Source: CAD feature listing. Evaluate the final solid. Frame: model axes, mm. A direction names the side the tool comes from. Coordinates: 2 decimals unless noted, no trailing zeros. Order: outer loops, then holes, each group sorted by start corner. A loop starts at its lowest first (then second) coordinate and runs counter-clockwise, first axis right, second up.
Item 1: Contact query for flat-ended pins moving along their axis: P1, Ø5.5, axis at x = -20, y = 0, coming from the -Z side; P2, Ø1, axis at y = 7.5, z = 121.5, coming from the -X side; P3, Ø5, axis at x = 9.5, z = 38.5, coming from the -Y side; P4, Ø2.5, axis at x = 0, y = 0, coming from the -Z side. Output: stop coordinate, or through.
Item 2: Ray query, line 1 (Y direction, x = 0, z = 12); line 2 (Z direction, x = 11, y = 11); line 3 (X direction, y = -20, z = 20). Return the intervals inside material, ascending.
Item 3: Reachability of faces 1 (the flat face through (0, -4, -14)), 2 (the flat face through (5, -5, 0)), 3 (the flat face through (0, 0, 191)) from +Z, -Z, +X, -X, +Y, -Y: full face, straight path, thin tool, end or side. Return the list, or none.
Item 4: Mould query, pull axis X, two halves, no side actions, for faces 4 (the conical face through (0.08, 19.64, 33.04)), 5 (the cylindrical face through (-20.633, -15.821, 94.181)), 6 (the flat face through (1, 1, -22)). Classes: released by +X, released by -X, zero draft, split by the parting line, or undercut.
Item 5: Section A-A on z = 11. Return the cut outline in (x, y).
Item 6: Section B-B on z = 46. Return the cut outline in (x, y), then the cut area to 3 significant figures.
from build123d import *

# Parameters (mm, degrees)
SKETCH1_R                 = 26
BODY_DEPTH                = 191
SKETCH2_R                 = 6
AXLE_DEPTH                = 22
FLAT_START                = -15
SKETCH3_R                 = 1.016
FLAT_DEPTH                = 15
M5X0_8_TAPPED_HOLE1_D     = 4.2
M5X0_8_TAPPED_HOLE1_DEPTH = 32.0000122
M5X0_8_TAPPED_HOLE1_TIP   = 1.2618073
FILLET1_R                 = 1.27


with BuildPart() as part:
    # Sketch1 → body (new body)
    with BuildSketch(Plane.XY):
        Circle(SKETCH1_R)
    extrude(amount=BODY_DEPTH)

    # Sketch2 → axle (add)
    with BuildSketch(Plane(origin=(0, 0, 0), x_dir=(-1, 0, 0), z_dir=(0, 0, -1))):
        with Locations(Location((0, 0, 0), (0, 0, 180))):
            Circle(SKETCH2_R)
    extrude(amount=AXLE_DEPTH)

    # Sketch3 → flat (cut)
    with BuildSketch(Plane(origin=(0, 0, -22), x_dir=(-1, 0, 0), z_dir=(0, 0, -1)).offset(FLAT_START)):
        with BuildLine():
            Line((4.472135955, -4), (-4.472135955, -4))
            ThreePointArc((-4.472135955, -4), (0, -6), (4.472135955, -4))
        make_face()
        Circle(SKETCH3_R)
    extrude(amount=FLAT_DEPTH, mode=Mode.SUBTRACT)

    # M5x0.8 Tapped Hole1
    with Locations(Plane(origin=(0, 0, 0), x_dir=(-1, 0, 0), z_dir=(0, 0, -1))):
        with Locations((0, -20), (-20, 0), (0, 20), (20, 0)):
            Hole(M5X0_8_TAPPED_HOLE1_D / 2, depth=M5X0_8_TAPPED_HOLE1_DEPTH)
            with Locations((0, 0, -(M5X0_8_TAPPED_HOLE1_DEPTH + M5X0_8_TAPPED_HOLE1_TIP / 2))):  # 118° drill point
                Cone(0, M5X0_8_TAPPED_HOLE1_D / 2, M5X0_8_TAPPED_HOLE1_TIP, mode=Mode.SUBTRACT)

    # Fillet1
    fillet1_edges = [part.edges().sort_by_distance(p)[0] for p in [
        (-26, 0, 0),
        (-26, 0, 191),
    ]]
    fillet(fillet1_edges, radius=FILLET1_R)


solid = part.part
Answer list:
1. P1: stops at z = 0
1. P2: stops at x = -25.04
1. P3: stops at y = -25.04
1. P4: stops at z = -22
2. line 1: y = -26 to -22.1, -17.9 to 17.9, 22.1 to 26
2. line 2: z = 0 to 191
2. line 3: x = -16.61 to -2.1, 2.1 to 16.61
3. face 1: -Z, +X, -X, -Y
3. face 2: -Z
3. face 3: +Z, +X, -X, +Y, -Y
4. face 4: undercut
4. face 5: split by the parting line
4. face 6: zero draft
5. outline: circle Ø52 at (0, 0); hole circle Ø4.2 at (-20, 0); hole circle Ø4.2 at (0, -20); hole circle Ø4.2 at (0, 20); hole circle Ø4.2 at (20, 0)
6. outline: circle Ø52 at (0, 0)
6. area: 2,120 mm2
